Could you check a few things on this model? Use its own coordinates, in mm. A direction names the side the tool comes from. Round coordinates to 2 decimals unless told otherwise and drop trailing zeros. Write each loop counter-clockwise with the first axis right and the second up, starting at its lowest first coordinate (ties: lowest second). Pieces come first, ordered by that corner, then holes. Notation, with made-up numbers: (37, 70.25) - (88, 70.25) arc R13 ccw to (88, 89.25) - close; hole circle Ø11 at (-8, 3.25). An arc over 180 degrees is marked (long way). Put each result on its own line as item: value.
from build123d import *

# Parameters (mm, degrees)
SKETCH_1_W               = 40
SKETCH_1_H               = 44
SKETCH_1_R               = 4.5
EXTRUDE_1_DEPTH          = 5
SKETCH_2_R               = 5.25
CUT_EXTRUDE_1_DEPTH      = 1
SKETCH_3_W               = 18
SKETCH_3_H               = 44
CUT_EXTRUDE_2_DEPTH      = 6
SKETCH_4_R               = 4.5
EXTRUDE_2_DEPTH          = 5
SKETCH_5_W               = 22
SKETCH_5_H               = 5
EXTRUDE_3_DEPTH          = 7
EXTRUDE_4_DEPTH          = 4
SKETCH_7_R               = 1.5
CUT_EXTRUDE_3_DEPTH      = 5
CUT_EXTRUDE_4_DEPTH      = 0.5
CUT_EXTRUDE_4_DEPTH_BACK = 2.5
EXTRUDE_5_DEPTH          = 5


with BuildPart() as part:
    # 草图1 → 凸台-拉伸1 (new body)
    with BuildSketch(Plane(origin=(0, 0, 0), x_dir=(0, 0, -1), z_dir=(1, 0, 0))):
        with Locations((9, -5)):
            Rectangle(SKETCH_1_W, SKETCH_1_H)
        Circle(SKETCH_1_R, mode=Mode.SUBTRACT)
        with Locations((18, 6)):
            Circle(SKETCH_1_R, mode=Mode.SUBTRACT)
        with Locations((11.543885882, -13.351449313)):
            Circle(SKETCH_1_R, mode=Mode.SUBTRACT)
    extrude(amount=EXTRUDE_1_DEPTH)

    # 草图2 → 切除-拉伸1 (cut)
    with BuildSketch(Plane.ZY.offset(-5)):
        with Locations((-18, 6)):
            Circle(SKETCH_2_R)
        Circle(SKETCH_2_R)
    extrude(amount=CUT_EXTRUDE_1_DEPTH, mode=Mode.SUBTRACT)

    # 草图3 → 切除-拉伸2 (cut, through all)
    with BuildSketch(Plane(origin=(5, 0, 0), x_dir=(0, 0, -1), z_dir=(1, 0, 0))):
        with Locations((-2, -5)):
            Rectangle(SKETCH_3_W, SKETCH_3_H)
    extrude(amount=-CUT_EXTRUDE_2_DEPTH, mode=Mode.SUBTRACT)

    # 草图4 → 凸台-拉伸2 (add, through all)
    with BuildSketch(Plane(origin=(5, 0, 0), x_dir=(0, 0, -1), z_dir=(1, 0, 0))):
        with Locations((11.543885882, -13.351449313)):
            Circle(SKETCH_4_R)
    extrude(amount=-EXTRUDE_2_DEPTH)

    # 草图5 → 凸台-拉伸3 (add)
    with BuildSketch(Plane(origin=(5, 0, 0), x_dir=(0, 0, -1), z_dir=(1, 0, 0))):
        with Locations((18, -24.5)):
            Rectangle(SKETCH_5_W, SKETCH_5_H)
    extrude(amount=EXTRUDE_3_DEPTH)

    # 草图6 → 凸台-拉伸4 (add)
    with BuildSketch(Plane.XZ.offset(27)):
        with BuildLine():
            Line((0, -29), (10, -29))
            ThreePointArc((10, -29), (12, -27), (10, -25))
            Line((10, -25), (0, -25))
            Line((0, -25), (0, -29))
        make_face()
    extrude(amount=EXTRUDE_4_DEPTH)

    # 草图7 → 切除-拉伸3 (cut)
    with BuildSketch(Plane.XZ.offset(27)):
        with Locations((6.5, -15)):
            Circle(SKETCH_7_R)
    extrude(amount=-CUT_EXTRUDE_3_DEPTH, mode=Mode.SUBTRACT)

    # 草图8 → 切除-拉伸4 (cut, two sides)
    with BuildSketch(Plane(origin=(0, -22, 0), x_dir=(-1, 0, 0), z_dir=(0, 1, 0))) as cut_extrude_4_sk:
        Polygon((-9.704293994, -15), (-8.102146997, -17.775), (-4.897853003, -17.775), (-3.295706006, -15), (-4.897853003, -12.225), (-8.102146997, -12.225), align=None)
    extrude(amount=CUT_EXTRUDE_4_DEPTH, mode=Mode.SUBTRACT)
    extrude(cut_extrude_4_sk.sketch, amount=-CUT_EXTRUDE_4_DEPTH_BACK, mode=Mode.SUBTRACT)

    # 草图9 → 凸台-拉伸5 (add)
    with BuildSketch(Plane(origin=(0, 0, -29), x_dir=(-1, 0, 0), z_dir=(0, 0, -1))):
        Polygon((-5, -22), (-12, -22), (-5, 0), align=None)
    extrude(amount=-EXTRUDE_5_DEPTH)


solid = part.part
(1) I'm going to push flat-ended pins straight in: pin 1 (3 mm diameter, centred on x = 5.5, z = -14, fed in from +Y); pin 2 (2 mm diameter, centred on y = 2.5, z = -9, fed in from +X); pin 3 (0.5 mm diameter, centred on x = 4.5, z = -15, fed in from -Y); pin 4 (2 mm diameter, centred on x = 4, y = -29, fed in from +Z). Where does each tip first touch, or does it pass through?
Values found:
pin 1: stops at y = 17
pin 2: stops at x = 5
pin 3: stops at y = -27
pin 4: stops at z = -25
(2) Please list where these lines run through material, in increasing order: probe 1 along Y at (x, z) = (4.4, -18); probe 2 along Z at (x, y) = (6.5, -25.35); probe 3 along Y at (x, z) = (2.85, -18). Write a range as from..to.
Values found:
probe 1: y = -27..0.75, 11.25..17
probe 2: z = -29..-16.5, -13.5..-7
probe 3: y = -27..1.5, 10.5..17
(3) If we mould it in two halves opening along X, with no side actions, what happens to faces 5 (the face through (8.914, -23.232, -16.368)), 6 (the face through (5, -2, -15)), 7 (the face through (3, -5, -7))? For each: pulls with the +X half, pulls with the -X half, needs draft (parallel to the pull), parting line crosses it, or undercut.
Values found:
face 5: undercut
face 6: pulls with the +X half
face 7: needs draft
(4) Imagine slicing it at C-C, the plane z = -19.5. List the corners of the cut face in (x, y) for me, then the cut area to 3 significant figures.
Values found:
outline: (0, -27) - (12, -27) - (12, -22) - (5, -22) - (5, 0.97) - (4, 0.97) - (4, 1.76) - (0, 1.76) - close; (0, 10.24) - (4, 10.24) - (4, 11.03) - (5, 11.03) - (5, 17) - (0, 17) - close
area: 211 mm^2
(5) Imagine slicing it at D-D, the plane x = 1.25. List the corners of the cut face in (y, z) for me.
Values found:
outline: (-31, -29) - (17, -29) - (17, -7) - (-27, -7) - (-27, -25) - (-31, -25) - close; hole circle Ø9 at (6, -18)
(6) For faces 1 (the face through (11.6, -27, -28.6)), 2 (the face through (5, -29, -25)), 3 (the face through (5, -24.5, -14)), 4 (the face through (7, -16, -24)), which set-ups out of +Z, -Z, +X, -X, +Y, -Y let a thin tool reach every point of the face, with its end or its side?
Values found:
face 1: -Z, +X, -Y
face 2: +Z, +X, -X, -Y
face 3: none
face 4: +Z, +X, +Y
(7) Imagine slicing it at A-A, the plane y = 6. List the corners of the cut face in (x, z) for me, then the cut area to 3 significant figures.
Values found:
outline: (0, -29) - (5, -29) - (5, -23.25) - (4, -23.25) - (4, -22.5) - (0, -22.5) - close; (0, -13.5) - (4, -13.5) - (4, -12.75) - (5, -12.75) - (5, -7) - (0, -7) - close
area: 63.5 mm^2
(8) Imagine slicing it at B-B, the plane x = 6. List the corners of the cut face in (y, z) for me (3 decimals), then the cut area to 3 significant figures.
Values found:
outline: (-31, -29) - (-3.143, -29) - (-3.143, -24) - (-22, -24) - (-22, -17.775) - (-24.5, -17.775) - (-24.5, -16.414) - (-27, -16.414) - (-27, -25) - (-31, -25) - close; (-27, -13.586) - (-24.5, -13.586) - (-24.5, -12.225) - (-22, -12.225) - (-22, -7) - (-27, -7) - close
area: 199 mm^2
